```python
from build123d import *

# Parameters (mm, degrees)
F0_R     = 175
F0_R_2   = 2
F0_W     = 5
F0_H     = 5
F1_DEPTH = 4


with BuildPart() as f1:
    # F0 (on Top) → F1 (new body)
    with BuildSketch(Plane.XY):
        Circle(F0_R)
        with Locations((-161.10979, -21.210506)):
            Circle(F0_R_2, mode=Mode.SUBTRACT)
        with Locations((21.210506, -161.10979)):
            Circle(F0_R_2, mode=Mode.SUBTRACT)
        with Locations((0, -60)):
            Rectangle(F0_W, F0_H, mode=Mode.SUBTRACT)
        with Locations((-60, 0)):
            Rectangle(F0_W, F0_H, mode=Mode.SUBTRACT)
        with Locations((-21.210506, 161.10979)):
            Circle(F0_R_2, mode=Mode.SUBTRACT)
        with Locations((60, 0)):
            Rectangle(F0_W, F0_H, mode=Mode.SUBTRACT)
        with Locations((0, 60)):
            Rectangle(F0_W, F0_H, mode=Mode.SUBTRACT)
        with Locations((161.10979, 21.210506)):
            Circle(F0_R_2, mode=Mode.SUBTRACT)
    extrude(amount=F1_DEPTH)


solid = f1.part
```
The listing builds one solid part. Answer for the finished solid, in the listing's coordinates (mm). Coordinates: 2 decimals unless noted, no trailing zeros. Write each loop counter-clockwise with the first axis right and the second up, starting at its lowest first coordinate (ties: lowest second). Pieces come first, ordered by that corner, then holes. Notation, with made-up numbers: M 33,-38 L 43,-38 A21 cw 43,-28 Z; hole C 11,46.25 d4. An arc over 180 degrees is marked long. Use a Markdown table: item, result. Add a question column.
1. Section B-B (y = 148.5) is taken. Give the vertices of the cut face in (x, z), plus the area to 3 significant figures.
2. Section C-C (y = -75) is taken. Give the vertices of the cut face in (x, z), plus the area to 3 significant figures.
3. Straight lines are drawn through the part: line 1 along X through (y, z) = (-5.5, 0.6); line 2 along Y through (x, z) = (20.5, 3.55); line 3 along X through (y, z) = (-37, 1.7). For each, find the intervals that lie inside material, in ascending order. Write a range as [from, to].
4. Section A-A (z = 0.8) is taken. Count the separate pieces of the cut face and the enclosed holes in it, plus the area to 3 significant figures.
5. Given P1, Ø2, axis at y = -60, z = 2, coming from the +X side; P2, Ø2, axis at x = 60.5, z = 1.5, coming from the -Y side; P3, Ø2, axis at x = -94.5, z = 1, coming from the -Y side; P4, Ø1.2, axis at y = 0.5, z = 1.5, coming from the +X side, each flat-ended and moving along its own axis, determine where each tip first touches the part or whether it passes through.
Data:
| question | item | result |
|---|---|---|
| 1 | outline | M -92.59,0 L 92.59,0 L 92.59,4 L -92.59,4 Z |
| 1 | area | 741 mm2 |
| 2 | outline | M -158.11,0 L 158.11,0 L 158.11,4 L -158.11,4 Z |
| 2 | area | 1,260 mm2 |
| 3 | line 1 | x = [-174.91, 174.91] |
| 3 | line 2 | y = [-173.8, -162.98], [-159.24, 173.8] |
| 3 | line 3 | x = [-171.04, 171.04] |
| 4 | separate pieces | 1 |
| 4 | enclosed holes | 8 |
| 4 | area | 96,100 mm2 |
| 5 | P1 | stops at x = 164.75 |
| 5 | P2 | stops at y = -164.57 |
| 5 | P3 | stops at y = -147.93 |
| 5 | P4 | stops at x = 175 |
